For this review, take the finished solid that the model builds, in its own axes (mm). A direction names the side the tool comes from. Round coordinates to 2 decimals unless told otherwise and drop trailing zeros. Write each loop counter-clockwise with the first axis right and the second up, starting at its lowest first coordinate (ties: lowest second). Pieces come first, ordered by that corner, then holes. Notation, with made-up numbers: (83, 32.25) - (95, 32.25) arc R25 ccw to (95, 62.25) - close; hole circle Ø1 at (19.5, 48). An arc over 180 degrees is marked (long way). One line per item, written item: value. Start each with the question number.
Q1. Add section B-B on y = 17. Write out the cut boundary in (x, z), and give its area (3 significant figures).
Q2. For probe 1 along X at (y, z) = (1, 14); probe 2 along Z at (x, y) = (-3.1, 17); probe 3 along X at (y, z) = (18.5, -15), list the stretches that pass through material, from the lowest coordinate up.
Q3. Add section D-D on x = 1. Write out the cut boundary in (y, z), and give its area (3 significant figures).
Q4. Clearance check with flat-ended pins moving along their axes: pin 1 Ø1.8 at (x, z) = (0, -14) entering from -Y; pin 2 Ø3.5 at (x, y) = (-3, 17) entering from +Z; pin 3 Ø3.5 at (x, z) = (0, -8.5) entering from +Y; pin 4 Ø1.5 at (x, z) = (1, -0.5) entering from +Y. State where each tip first meets the part, or that it passes through.
Q5. Add section C-C on x = -4.75. Write out the cut boundary in (y, z), and give its area (3 significant figures).
Q6. Add section A-A on z = 14. Write out the cut boundary in (x, y).
Q7. Mouldability with a two-part tool opening along X and no side actions: class faces 1 (the face through (5, 1, -19)), 2 (the face through (-2, 15, -20)), 3 (the face through (-1.464, 1.642, -14.325)) as +X half, -X half, draft (parallel to the pull), parting line (faces both ways), or undercut.
Q8. Tool access review of faces 4 (the face through (-1.2, 3.8, -0.7)), 5 (the face through (-4, 15, 10)), 6 (the face through (-3.98, 6.26, -1.62)): name each direction out of +Z, -Z, +X, -X, +Y, -Y from which nothing blocks a thin tool from reaching the whole face with its end or side.
```python
from build123d import *

# Parameters (mm, degrees)
SKETCH1_R                = 1.5
BOSS_EXTRUDE1_DEPTH      = 3
BOSS_EXTRUDE2_DEPTH      = 28
CHAMFER1_SIZE            = 2
SKETCH4_R                = 11
CUT_EXTRUDE1_DEPTH       = 11
CHAMFER2_SIZE            = 6
CHAMFER2_OF_MIRROR3_SIZE = 6
CHAMFER3_SIZE            = 2
SKETCH5_W                = 30
SKETCH5_H                = 28
CUT_EXTRUDE2_DEPTH       = 11
CHAMFER4_SIZE            = 1.5


with BuildPart() as part:
    # Sketch1 → Boss-Extrude1 (new body)
    with BuildSketch(Plane(origin=(0, 0, 0), x_dir=(1, 0, 0), z_dir=(0, 1, 0))):
        Polygon((-6, 20), (6, 20), (6, -17), (3, -20), (-3, -20), (-6, -17), align=None)
        with Locations(Location((0, 14, 0), (0, 0, 270))):
            Circle(SKETCH1_R, mode=Mode.SUBTRACT)
        with Locations(Location((0, -14, 0), (0, 0, 270))):
            Circle(SKETCH1_R, mode=Mode.SUBTRACT)
    extrude(amount=BOSS_EXTRUDE1_DEPTH)

    # Sketch2 → Boss-Extrude2 (add)
    with BuildSketch(Plane(origin=(0, 3, 0), x_dir=(1, 0, 0), z_dir=(0, 1, 0))):
        Polygon((6, -10), (6, 20), (0.1, 20), (1.9, 15.9), (1.9, -10), align=None)
    boss_extrude2 = extrude(amount=BOSS_EXTRUDE2_DEPTH)

    # Chamfer1
    chamfer1_edges = [part.edges().sort_by_distance(p)[0] for p in [
        (6, 15.5, -20),
    ]]
    chamfer(chamfer1_edges, length=CHAMFER1_SIZE)

    # Sketch4 → Cut-Extrude1 (cut)
    with BuildSketch(Plane(origin=(6, 0, 0), x_dir=(0, 0, -1), z_dir=(1, 0, 0))):
        with Locations((4, 17)):
            Circle(SKETCH4_R)
    cut_extrude1 = extrude(amount=-CUT_EXTRUDE1_DEPTH, mode=Mode.SUBTRACT)

    # Chamfer2
    chamfer2_edges = [part.edges().sort_by_distance(p)[0] for p in [
        (3.95, 31, 10),
    ]]
    chamfer(chamfer2_edges, length=CHAMFER2_SIZE)

    # Mirror3: Boss-Extrude2, Cut-Extrude1 across plane
    add(boss_extrude2.mirror(Plane(origin=(0, 0, 0), x_dir=(0, 0, 1), z_dir=(1, 0, 0))))
    add(cut_extrude1.mirror(Plane(origin=(0, 0, 0), x_dir=(0, 0, 1), z_dir=(1, 0, 0))), mode=Mode.SUBTRACT)

    # Chamfer2 of Mirror3
    chamfer2_of_mirror3_edges = [part.edges().sort_by_distance(p)[0] for p in [
        (-3.95, 31, 10),
    ]]
    chamfer(chamfer2_of_mirror3_edges, length=CHAMFER2_OF_MIRROR3_SIZE)

    # Chamfer3
    chamfer3_edges = [part.edges().sort_by_distance(p)[0] for p in [
        (-6, 15.5, -20),
    ]]
    chamfer(chamfer3_edges, length=CHAMFER3_SIZE)

    # Sketch5 → Cut-Extrude2 (cut)
    with BuildSketch(Plane(origin=(0, 0, 0), x_dir=(0, 0, -1), z_dir=(1, 0, 0))):
        with Locations((5, 17)):
            Rectangle(SKETCH5_W, SKETCH5_H)
    extrude(amount=CUT_EXTRUDE2_DEPTH, mode=Mode.SUBTRACT)

    # Chamfer4
    # the kernel refuses this chamfer: 1.5 mm, written as the material it adds along each edge
    with BuildSketch(Plane(origin=(-1.9, 3, 10), x_dir=(0, -0.02749587661058648, 0.9996219169112968), z_dir=(-1, 0, 0))) as chamfer4_piece_1:
        Polygon((CHAMFER4_SIZE * 0.999621916911, CHAMFER4_SIZE * 0.0274958766106), (-CHAMFER4_SIZE * 0.0274958766106, CHAMFER4_SIZE * 0.999621916911), (0, 0), align=None)
    extrude(amount=4.1)
    with BuildSketch(Plane(origin=(-1.9, 3, -19.757524482), x_dir=(-0.02749587661058635, 0.9996219169112968, 0), z_dir=(0, 0, 1))) as chamfer4_piece_2_section:
        Polygon((CHAMFER4_SIZE * 0.999621916911, -CHAMFER4_SIZE * 0.0274958766106), (-CHAMFER4_SIZE * 0.0274958766106, -CHAMFER4_SIZE * 0.999621916911), (0, 0), align=None)
    chamfer4_piece_2 = extrude(amount=29.757524482, mode=Mode.PRIVATE)
    chamfer4_piece_2 = chamfer4_piece_2 - Plane(origin=(0, 3.558405008, -14), x_dir=(0, 0, 1), z_dir=(0, -1, 0)) * Cylinder(1.5, 66, mode=Mode.PRIVATE)
    add(chamfer4_piece_2)
    with BuildSketch(Plane(origin=(-1.9, 3, -19.757524482), x_dir=(-0.02749587661058635, 0.9996219169112968, 0), z_dir=(0, 0, 1))) as chamfer4_piece_3a_section:
        Polygon((CHAMFER4_SIZE * 0.999621916911, -CHAMFER4_SIZE * 0.0274958766106), (-CHAMFER4_SIZE * 0.0274958766106, -CHAMFER4_SIZE * 0.999621916911), (0, 0), align=None)
    chamfer4_piece_3a = extrude(amount=33.615048964, mode=Mode.PRIVATE)
    chamfer4_piece_3a = split(chamfer4_piece_3a, bisect_by=Plane(origin=(-1.452850979, 3.51967463, 10), z_dir=(0, 0, 1)), keep=Keep.TOP, mode=Mode.PRIVATE)
    chamfer4_piece_3a = chamfer4_piece_3a - Plane(origin=(0, 3.51967463, 14), x_dir=(0, 0, 1), z_dir=(0, -1, 0)) * Cylinder(1.5, 74, mode=Mode.PRIVATE)
    with BuildSketch(Plane(origin=(1.957524482, 3, 10), x_dir=(0, -0.02749587661058648, 0.9996219169112968), z_dir=(-1, 0, 0))) as chamfer4_piece_3b_section:
        Polygon((CHAMFER4_SIZE * 0.999621916911, CHAMFER4_SIZE * 0.0274958766106), (-CHAMFER4_SIZE * 0.0274958766106, CHAMFER4_SIZE * 0.999621916911), (0, 0), align=None)
    chamfer4_piece_3b = extrude(amount=7.957524482, mode=Mode.PRIVATE)
    chamfer4_piece_3b = split(chamfer4_piece_3b, bisect_by=Plane(origin=(-1.9, 3.49469044, 10.49469044), z_dir=(1, 0, 0)), keep=Keep.TOP, mode=Mode.PRIVATE)
    chamfer4_piece_3 = chamfer4_piece_3a & chamfer4_piece_3b
    add(chamfer4_piece_3)


solid = part.part
```
Result set:
1. outline: (-6, -18) - (-4, -20) - (-0.1, -20) - (-1.9, -15.9) - (-1.9, -15) - (-6, -15) - close; (-6, 7) - (-1.9, 7) - (-1.9, 10) - (-6, 10) - close
1. area: 34.5 mm^2
2. probe 1: x = -6 to -1.5, 1.5 to 6
2. probe 2: z = -20 to -15, 7 to 10
2. probe 3: x = -6 to -1.9
3. outline: (0, -20) - (3, -20) - (3, -15.12) - (0, -15.12) - close; (0, -12.88) - (3, -12.88) - (3, 12.88) - (0, 12.88) - close; (0, 15.12) - (3, 15.12) - (3, 20) - (0, 20) - close
3. area: 107 mm^2
4. pin 1: passes through
4. pin 2: stops at z = 10
4. pin 3: stops at y = 4.35
4. pin 4: stops at y = 3
5. outline: (0, -19.25) - (31, -19.25) - (31, 4) - (25, 10) - (4.5, 10) - (3, 11.5) - (3, 18.25) - (0, 18.25) - close; hole circle Ø22 at (17, -4)
5. area: 534 mm^2
6. outline: (-6, 0) - (-1.5, 0) - (-1.5, 3) - (-6, 3) - close; (1.5, 0) - (6, 0) - (6, 3) - (1.5, 3) - close
7. face 1: +X half
7. face 2: draft
7. face 3: undercut
8. face 4: +Z, +X, +Y
8. face 5: +Z, +X, -X, +Y
8. face 6: +X, -X
